Here's how the part is built. I have some questions about the finished solid (model axes, mm). Give positions to 0.01 mm unless a question says otherwise; leave off trailing zeros. Write each loop counter-clockwise with the first axis right and the second up, starting at its lowest first coordinate (ties: lowest second). Pieces come first, ordered by that corner, then holes. Notation, with made-up numbers: (33, -11.5) - (89, -11.5) arc R28 ccw to (89, 17.5) - close; hole circle Ø3 at (72.5, -32). An arc over 180 degrees is marked (long way). Use a Markdown table: item, result.
Autodesk Inventor part; units mm, degrees
ref_plane "YZ Plane" through (0, 0, 0) normal (1, 0, 0) x (0, 1, 0)
ref_plane "XZ Plane" through (0, 0, 0) normal (0, 1, 0) x (-1, 0, 0)
ref_plane "XY Plane" through (0, 0, 0) normal (0, 0, 1) x (1, 0, 0)
sketch "Sketch1" plane through (0, 0, 0) normal (0, 1, 0) x (-1, 0, 0)
  circle A0 centre (130.175, -139.7) radius 3.3782
  circle A1 centre (130.175, -28.4093) radius 3.3782
  line L0 (146.05, 23.2231) -> (123.825, -22.0593)
  line L1 (123.825, -22.0593) -> (123.825, -146.05)
  line L2 (123.825, -146.05) -> (146.05, -146.05)
  line L3 (146.05, -146.05) -> (146.05, 23.2231)
  point P0 (0, 0)
  point P1 (0, 0)
  dimension "d0" = 22.225
extrude "Extrusion1" add sketch "Sketch1" along normal blind 6.35
properties part number "Spacer"
Item 1: I need wall thicknesses on line 1 along X through (y, z) = (2.5, -139.7) (3 decimals); line 2 along Z through (x, y) = (-131.5, 6.25); line 3 along Z through (x, y) = (-133, 4.75). Which ranges of each line are inside material? Lowest first, please. Write a range as [from, to].
Values:
| item | result |
|---|---|
| line 1 | x = [-146.05, -133.553], [-126.797, -123.825] |
| line 2 | z = [-146.05, -142.81], [-136.59, -31.52], [-25.3, -6.42] |
| line 3 | z = [-146.05, -141.55], [-137.85, -30.26], [-26.56, -3.37] |
Item 2: Will this pin go through, and if not, where does the flat tip stop? pin 1 Ø5.5 at (x, z) = (-130.18, -28.41) entering from +Y.
Values:
| item | result |
|---|---|
| pin 1 | passes through |
Item 3: Thinking about a two-plate mould opening in Z: for faces 1 (the flat face through (-146.05, 3, -63)), 2 (the flat face through (-135, 3, -146.05)), 3 (the cylindrical face through (-133.4, 3.1, -140.7)), which applies, +Z half, -Z half, draft (parallel to the pull), parting line (faces both ways), or undercut?
Values:
| item | result |
|---|---|
| face 1 | draft |
| face 2 | -Z half |
| face 3 | undercut |
Item 4: If we section it at B-B, the plane x = -129.75: Write out the boundary of the cut face in (y, z).
Values:
| item | result |
|---|---|
| outline | (0, -146.05) - (6.35, -146.05) - (6.35, -143.05) - (0, -143.05) - close; (0, -136.35) - (6.35, -136.35) - (6.35, -31.76) - (0, -31.76) - close; (0, -25.06) - (6.35, -25.06) - (6.35, -9.99) - (0, -9.99) - close |
Item 5: If we section it at A-A, the plane z = -139.7: Write out the boundary of the cut face in (x, y) (3 decimals), plus the area to 3 significant figures.
Values:
| item | result |
|---|---|
| outline | (-146.05, 0) - (-133.553, 0) - (-133.553, 6.35) - (-146.05, 6.35) - close; (-126.797, 0) - (-123.825, 0) - (-123.825, 6.35) - (-126.797, 6.35) - close |
| area | 98.2 mm2 |
Item 6: If we section it at D-D, the plane z = -13: Write out the boundary of the cut face in (x, y).
Values:
| item | result |
|---|---|
| outline | (-146.05, 0) - (-128.27, 0) - (-128.27, 6.35) - (-146.05, 6.35) - close |
Item 7: If we section it at C-C, the plane y = 1: Write out the boundary of the cut face in (x, z) (3 decimals), plus the area to 3 significant figures.
Values:
| item | result |
|---|---|
| outline | (-146.05, -146.05) - (-123.825, -146.05) - (-123.825, -22.059) - (-146.05, 23.223) - close; hole circle Ø6.756 at (-130.175, -139.7); hole circle Ø6.756 at (-130.175, -28.409) |
| area | 3,190 mm2 |
